Geometry: see drawing. Coordinates: mm, zero at the bounding-box minimum. Coordinates: 2 decimals unless noted, no trailing zeros. Loops run counter-clockwise (first coordinate to the right, second up) from the corner with the lowest first, then second, coordinate; pieces in that order, holes last. Notation, with made-up numbers: (79, 40.5) -> (114, 40.5) arc R18 ccw to (114, 68.5) -> close; hole circle Ø2 at (-35, 57). An arc over 180 degrees is marked (long way). One line per item, written item: value. Start each with the question number.
Item 1: Section query D-D on z = 3. Return loops of the section in (x, y) (3 decimals).
Item 2: Section query B-B on y = 279.4. Return loops of the section in (x, z) (3 decimals).
Item 3: Section query C-C on x = 2.1. Return loops of the section in (y, z) (3 decimals), then the cut area to 3 significant figures.
Item 4: Section query A-A on z = 19.05. Return loops of the section in (x, y) (3 decimals).
Item 5: Ray query, probe 1 along Y at (x, z) = (2.75, 17.5); probe 2 along Z at (x, y) = (1.55, 12.7) (3 decimals); probe 3 along Y at (x, z) = (1.35, 21). Return the intervals inside material, ascending. Write a range as from..to.
Item 6: Contact query for flat-ended pins moving along their axis: pin 1 Ø1.5 at (x, z) = (1.5, 24) entering from -Y; pin 2 Ø1.5 at (x, z) = (1.5, 28) entering from -Y. Output: stop coordinate, or through.
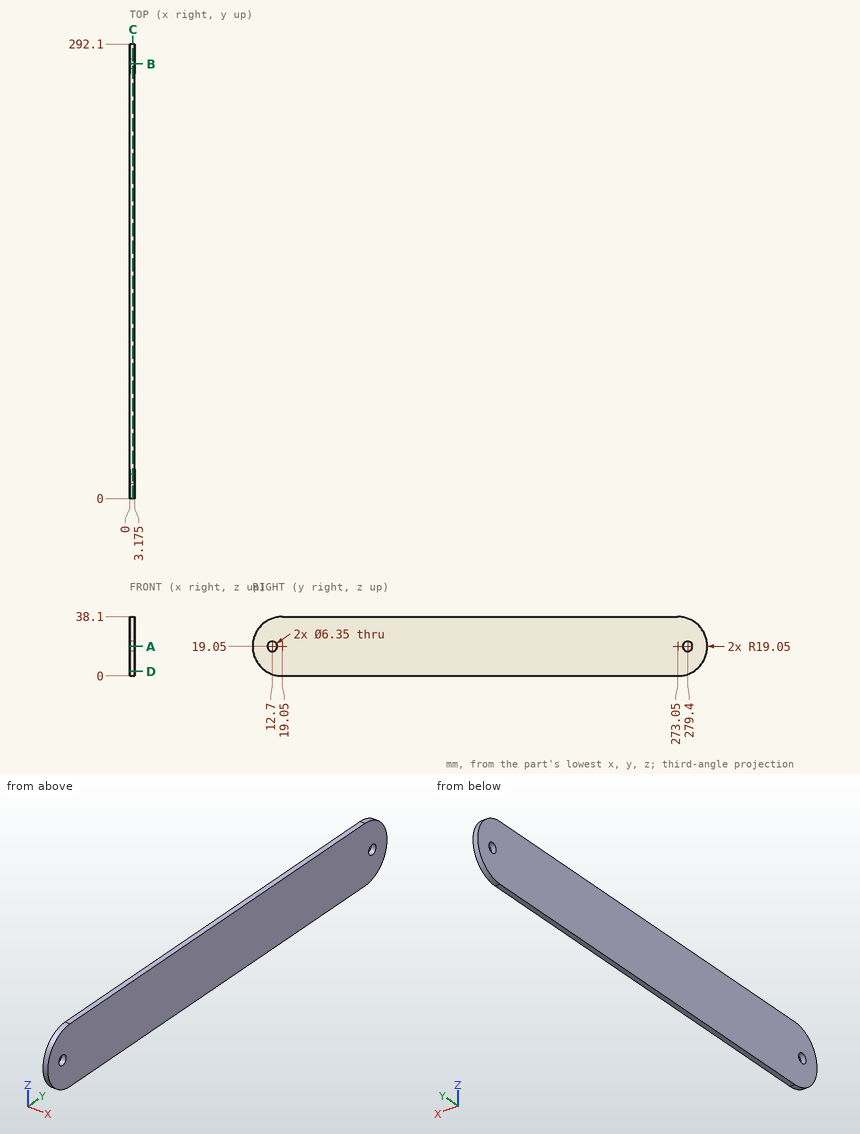
Reply:
1. outline: (0, 8.788) -> (3.175, 8.788) -> (3.175, 283.312) -> (0, 283.312) -> close
2. outline: (0, 1.089) -> (3.175, 1.089) -> (3.175, 15.875) -> (0, 15.875) -> close; (0, 22.225) -> (3.175, 22.225) -> (3.175, 37.011) -> (0, 37.011) -> close
3. outline: (19.05, 0) -> (273.05, 0) arc R19.05 ccw to (273.05, 38.1) -> (19.05, 38.1) arc R19.05 ccw to start; hole circle Ø6.35 at (12.7, 19.05); hole circle Ø6.35 at (279.4, 19.05)
3. area: 10,800 mm²
4. outline: (0, 0) -> (3.175, 0) -> (3.175, 9.525) -> (0, 9.525) -> close; (0, 15.875) -> (3.175, 15.875) -> (3.175, 276.225) -> (0, 276.225) -> close; (0, 282.575) -> (3.175, 282.575) -> (3.175, 292.1) -> (0, 292.1) -> close
5. probe 1: y = 0.06..9.93, 15.47..276.63, 282.17..292.04
5. probe 2: z = 1.089..15.875, 22.225..37.011
5. probe 3: y = 0.1..10.19, 15.21..276.89, 281.91..292
6. pin 1: stops at y = 0.47
6. pin 2: stops at y = 1.86
